Design review of the part built by this model. Coordinates are the model's own, in mm. A direction names the side the tool comes from. Coordinates: 2 decimals unless noted, no trailing zeros. Write each loop counter-clockwise with the first axis right and the second up, starting at its lowest first coordinate (ties: lowest second). Pieces come first, ordered by that corner, then holes. Notation, with made-up numbers: (50.5, 1.25) - (55.5, 1.25) arc R36 ccw to (55.5, 40.25) - close; hole circle Ø10 at (44.25, 74.5). An arc over 180 degrees is marked (long way). Use a Markdown table: item, result.
from build123d import *

# Parameters (mm, degrees)
RESSALTO_EXTRUS_O1_DEPTH = 62
FILETE1_R                = 0.2
ESBO_O3_R                = 1.0922
CORTE_EXTRUS_O1_DEPTH    = 5
CORTE_EXTRUS_O2_START    = -5
ESBO_O2_R                = 1.0922
CORTE_EXTRUS_O2_DEPTH    = 5


with BuildPart() as part:
    # Esboço1 → Ressalto-extrusão1 (new body)
    with BuildSketch(Plane(origin=(0, 0, 0), x_dir=(1, 0, 0), z_dir=(0, 1, 0))):
        Polygon((2.886751346, 0), (1.443375673, 2.5), (-1.443375673, 2.5), (-2.886751346, 0), (-1.443375673, -2.5), (1.443375673, -2.5), align=None)
    extrude(amount=RESSALTO_EXTRUS_O1_DEPTH)

    # Filete1
    filete1_edges = [part.edges().sort_by_distance(p)[0] for p in [
        (0, 62, -2.5),
        (-2.165063509, 62, -1.25),
        (-2.165063509, 62, 1.25),
        (0, 62, 2.5),
        (2.165063509, 62, 1.25),
        (0, 0, 2.5),
        (-2.165063509, 0, 1.25),
        (-2.165063509, 0, -1.25),
        (2.165063509, 62, -1.25),
        (0, 0, -2.5),
        (2.165063509, 0, -1.25),
        (2.165063509, 0, 1.25),
    ]]
    fillet(filete1_edges, radius=FILETE1_R)

    # Esboço3 → Corte-extrusão1 (cut)
    with BuildSketch(Plane(origin=(0, 62, 0), x_dir=(1, 0, 0), z_dir=(0, 1, 0))):
        with Locations(Location((0, 0, 0), (0, 0, 270))):
            Circle(ESBO_O3_R)
    extrude(amount=-CORTE_EXTRUS_O1_DEPTH, mode=Mode.SUBTRACT)

    # Esboço2 → Corte-extrusão2 (cut)
    with BuildSketch(Plane.XZ.offset(CORTE_EXTRUS_O2_START)):
        with Locations(Location((0, 0, 0), (0, 0, 90))):
            Circle(ESBO_O2_R)
    extrude(amount=CORTE_EXTRUS_O2_DEPTH, mode=Mode.SUBTRACT)


solid = part.part
(1) For pin 1 (1 mm diameter, centred on y = 29, z = -1, fed in from +X); pin 2 (1.7 mm diameter, centred on x = 0, z = 0, fed in from +Y); pin 3 (3 mm diameter, centred on y = 42, z = -1, fed in from -X), all flat-tipped, find the tip position at first contact; note any pin that passes through.
Determined:
| item | result |
|---|---|
| pin 1 | x = 2.6 |
| pin 2 | y = 57 |
| pin 3 | x = -2.89 |
(2) Draft analysis for pull direction X (two halves, no side actions). For faces 4 (the flat face through (0, 31, 2.5)), 5 (the cylindrical face through (0.33, 59.54, 1.04)), 6 (the flat face through (2.155, 30.569, 1.267)), state which applies: +X half, -X half, draft (parallel to the pull), parting line (faces both ways), or undercut.
Determined:
| item | result |
|---|---|
| face 4 | draft |
| face 5 | undercut |
| face 6 | +X half |
(3) Machinability: for faces 1 (the cylindrical face through (2.106, 61.94, -1.239)), 2 (the flat face through (0, 57, 0)), 3 (the flat face through (0, 5, 0)), which of the approach directions +Z, -Z, +X, -X, +Y, -Y give a long, thin tool a straight path to every point of the face, cutting with its end or side? Answer none if there is none.
Determined:
| item | result |
|---|---|
| face 1 | -Z, +X, +Y |
| face 2 | +Y |
| face 3 | -Y |
(4) For L1, parallel to X at y = 2.8, z = 0; L2, parallel to X at y = 44, z = 0.4; L3, parallel to Y at x = -0.65, z = -0.55, list the stretches that pass through material, from the lowest coordinate up. Write a range as from..to.
Determined:
| item | result |
|---|---|
| L1 | -2.89..-1.09, 1.09..2.89 |
| L2 | -2.66..2.66 |
| L3 | 5..57 |
(5) Take a section at A-A on x = 0. Write out the cut boundary in (y, z).
Determined:
| item | result |
|---|---|
| outline | (0, -2.3) arc R0.2 ccw to (0.2, -2.5) - (61.8, -2.5) arc R0.2 ccw to (62, -2.3) - (62, -1.09) - (57, -1.09) - (57, 1.09) - (62, 1.09) - (62, 2.3) arc R0.2 ccw to (61.8, 2.5) - (0.2, 2.5) arc R0.2 ccw to (0, 2.3) - (0, 1.09) - (5, 1.09) - (5, -1.09) - (0, -1.09) - close |
(6) Take a section at B-B on y = 34.5. Write out the cut boundary in (x, z), and give its area (3 significant figures).
Determined:
| item | result |
|---|---|
| outline | (-2.89, 0) - (-1.44, -2.5) - (1.44, -2.5) - (2.89, 0) - (1.44, 2.5) - (-1.44, 2.5) - close |
| area | 21.7 mm2 |
